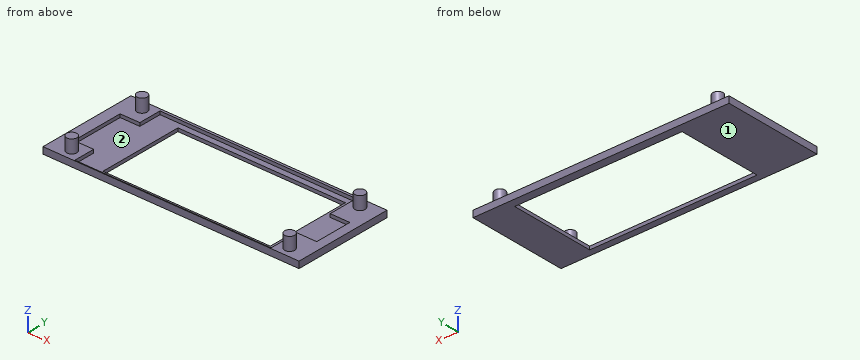
```python
from build123d import *

# Parameters (mm, degrees)
SKETCH_W        = 78
SKETCH_H        = 30.5
PAD_DEPTH       = 2
SKETCH002_W     = 51
SKETCH002_H     = 26
POCKET_DEPTH    = 5
POCKET001_DEPTH = 1
SKETCH001_R     = 1.55
PAD001_DEPTH    = 4


with BuildPart() as part:
    # Sketch → Pad (new body)
    with BuildSketch(Plane.XY):
        with Locations((0, 0.25)):
            Rectangle(SKETCH_W, SKETCH_H)
    extrude(amount=PAD_DEPTH)

    # Sketch002 (on Face6 of Pad) → Pocket (cut)
    with BuildSketch(Plane.XY.offset(2)):
        with Locations((3, 0)):
            Rectangle(SKETCH002_W, SKETCH002_H)
    extrude(amount=-POCKET_DEPTH, mode=Mode.SUBTRACT)

    # Sketch003 (on Face5 of Pocket) → Pocket001 (cut)
    with BuildSketch(Plane.XY.offset(2)):
        Polygon((-35.5, 7.75), (-35.5, -8.25), (-29.5, -8.25), (-29.5, -14.75), (30.25, -14.75), (30.25, -5.75), (36.25, -5.75), (36.25, 5.75), (30.25, 5.75), (30.25, 14.75), (-29.5, 14.75), (-29.5, 7.75), align=None)
    extrude(amount=-POCKET001_DEPTH, mode=Mode.SUBTRACT)

    # Sketch001 (on Face5 of Pocket) → Pad001 (join)
    with BuildSketch(Plane.XY.offset(2)):
        with Locations((33.5, 12.4)):
            Circle(SKETCH001_R)
        with Locations((33.5, -12)):
            Circle(SKETCH001_R)
        with Locations((-32.9, 12.4)):
            Circle(SKETCH001_R)
        with Locations((-32.9, -12)):
            Circle(SKETCH001_R)
    extrude(amount=PAD001_DEPTH)


solid = part.part
```
Check sheet for the modelled part. Datum: model origin and axes. Units: mm. Face numbers are marked on the shaded views. Coordinates: 2 decimals unless noted, no trailing zeros. Order: outer loops, then holes, each group sorted by start corner. A loop starts at its lowest first (then second) coordinate and runs counter-clockwise, first axis right, second up. Notation, with made-up numbers: M 14.25,62 L 73.25,62 A15 ccw 73.25,82 Z; hole C 77.25,-4 d9. An arc over 180 degrees is marked long. Write each question's results on one line, items separated by ' | '. Start each with the question number.
1. Go/stop test with flat-tipped pins: P1, Ø2, axis at x = -22, y = 1, coming from the +Z side; P2, Ø15, axis at x = 16, y = -4, coming from the +Z side (3 decimals); P3, Ø3, axis at x = -30.5, z = 5, coming from the +Y side. Record where each tip stops, or that it passes through.
2. Mould release check, pull along X, two halves, no side actions. Record for the marked faces 1 and 2: +X half, -X half, draft (parallel to the pull), parting line (faces both ways), or undercut.
3. Cross-section at B-B on y = -2. Record the cut outline in (x, z), and give its area (4 significant figures).
4. Cross-section at C-C on x = -32.9. Record the cut outline in (y, z).
5. Cross-section at D-D on z = 3.55. Record the cut outline in (x, y), and give its area (3 significant figures).
6. Cross-section at A-A on x = -6. Record the cut outline in (y, z), and give its area (3 significant figures).
7. Material ranges on probe 1 along Y at (x, z) = (-19, 1.9); probe 2 along X at (y, z) = (7, 0.3); probe 3 along X at (y, z) = (3.5, 1.65), recorded low to high.
Checks:
1) P1: stops at z = 1 | P2: passes through | P3: stops at y = 13.66
2) face 1: draft | face 2: undercut
3) outline: M -39,0 L -22.5,0 L -22.5,1 L -35.5,1 L -35.5,2 L -39,2 Z; M 28.5,0 L 39,0 L 39,2 L 36.25,2 L 36.25,1 L 28.5,1 Z | area: 33.25 mm²
4) outline: M -15,0 L 15.5,0 L 15.5,2 L 13.95,2 L 13.95,6 L 10.85,6 L 10.85,2 L 7.75,2 L 7.75,1 L -8.25,1 L -8.25,2 L -10.45,2 L -10.45,6 L -13.55,6 L -13.55,2 L -15,2 Z
5) outline: C -32.9,-12 d3.1; C -32.9,12.4 d3.1; C 33.5,-12 d3.1; C 33.5,12.4 d3.1 | area: 30.2 mm²
6) outline: M -15,0 L -13,0 L -13,1 L -14.75,1 L -14.75,2 L -15,2 Z; M 13,0 L 15.5,0 L 15.5,2 L 14.75,2 L 14.75,1 L 13,1 Z | area: 5.50 mm²
7) probe 1: y = -15 to -14.75, 14.75 to 15.5 | probe 2: x = -39 to -22.5, 28.5 to 39 | probe 3: x = -39 to -35.5, 36.25 to 39
